Autodesk Inventor part; units mm, degrees
ref_plane "YZ Plane" through (0, 0, 0) normal (1, 0, 0) x (0, 1, 0)
ref_plane "XZ Plane" through (0, 0, 0) normal (0, 1, 0) x (-1, 0, 0)
ref_plane "XY Plane" through (0, 0, 0) normal (0, 0, 1) x (1, 0, 0)
sketch "Sketch1" plane through (0, 0, 0) normal (0, 1, 0) x (-1, 0, 0)
  line L0 (10, 22.5) -> (-10, 22.5)
  line L1 (-10, 22.5) -> (-10, -22.5)
  line L2 (-10, -22.5) -> (10, -22.5)
  line L3 (10, -22.5) -> (10, 22.5)
  line L4 (10, 22.5) -> (-10, -22.5) construction
  line L5 (-10, 22.5) -> (10, -22.5) construction
  line L6 (13.4184, 10.4917) -> (6.5816, 10.4917)
  line L7 (6.5816, 10.4917) -> (6.5816, -10.4917)
  line L8 (6.5816, -10.4917) -> (13.4184, -10.4917)
  line L9 (13.4184, -10.4917) -> (13.4184, 10.4917)
  line L10 (13.4184, 10.4917) -> (6.5816, -10.4917) construction
  line L11 (6.5816, 10.4917) -> (13.4184, -10.4917) construction
  line L12 (8.5, 21) -> (-8.5, 21)
  line L13 (-8.5, 21) -> (-8.5, -21)
  line L14 (-8.5, -21) -> (8.5, -21)
  line L15 (8.5, -21) -> (8.5, 21)
  line L16 (8.5, 21) -> (-8.5, -21) construction
  line L17 (-8.5, 21) -> (8.5, -21) construction
  circle A0 centre (8.5, 21) radius 0.75
  circle A1 centre (8.5, -21) radius 0.75
  circle A2 centre (-8.5, -21) radius 0.75
  circle A3 centre (-8.5, 21) radius 0.75
  point P0 (0, 0)
  point P1 (10, 0)
  point P2 (10, 10.4917)
  point P3 (10, -10.4917)
  dimension "d0" = 20
  dimension "d1" = 45
  dimension "d2" = 17
  dimension "d3" = 42
  dimension "d4" = 1.5
  dimension "d5" = 1.5
  dimension "d6" = 1.5
  dimension "d7" = 1.5
extrude "Extrusion1" add sketch "Sketch1" along normal blind 2 contours L3 L6 L15 A0 L12 A3 L13 A2 L14 A1 L8 L2 L1 L0 | L6 L7 L8 L15 A1 L14 A2 L13 A3 L12 A0
sketch "Sketch2" plane through (0, 0, 0) normal (0, -1, 0) x (1, 0, 0)
  line L0 (10, -22.5) -> (-10, -22.5)
  line L1 (10, -22.5) -> (13, -22.5)
  line L2 (13, -22.5) -> (13, 22.5)
  line L3 (-10, 22.5) -> (10, 22.5)
  line L4 (13, 22.5) -> (10, 22.5)
  line L5 (10, 22.5) -> (10, -22.5)
  point P0 (0, 0)
  dimension "d10" = 3
  dimension "d11" = 45
extrude "Extrusion2" add sketch "Sketch2" along normal blind 10 and the other way blind 2
fillet "Fillet1" radius 2 1 edges at (10, 0, 0)
sketch "Sketch3" plane through (13, -10, 22.5) normal (1, 0, 0) x (0, 0, -1)
  line L0 (0, 0) -> (45, 0)
  line L1 (22.5, 0) -> (22.5, 5)
  line L2 (22.5, 5) -> (22.5, 6)
  line L3 (22.5, 6) -> (7.5, 6)
  line L4 (7.5, 6) -> (37.5, 6)
  circle A0 centre (37.5, 6) radius 1.5
  circle A1 centre (7.5, 6) radius 1.5
  point P0 (22.5, 10)
  dimension "d17" = 5
  dimension "d18" = 1
  dimension "d19" = 15
  dimension "d20" = 30
  dimension "d21" = 3
  dimension "d22" = 3
extrude "Extrusion3" cut sketch "Sketch3" against normal blind 10
properties part number "Ultrasonic_holder"
Work out the finished part from the listing and answer in its coordinate system (mm). A direction names the side the tool comes from. Coordinates: 2 decimals unless noted, no trailing zeros. Order: outer loops, then holes, each group sorted by start corner. A loop starts at its lowest first (then second) coordinate and runs counter-clockwise, first axis right, second up. Notation, with made-up numbers: M -16.5,40 L 22.5,40 A9 cw 22.5,47 Z; hole C 39,-31 d4. An arc over 180 degrees is marked long. Use CSV: the item, a comma, the result in double quotes.
1) Flat-ended cylindrical pins translate along their axes: pin 1 Ø1.4 at (x, z) = (-8.5, -21) entering from +Y; pin 2 Ø6 at (y, z) = (-1.5, 14) entering from -X; pin 3 Ø5 at (y, z) = (-6, 3.5) entering from -X; pin 4 Ø2 at (y, z) = (0.5, 3.5) entering from -X. Find the tip coordinate at first contact, or state that the pin passes through.
Worked out:
pin 1,"passes through"
pin 2,"stops at x = -10"
pin 3,"stops at x = 10"
pin 4,"stops at x = -6.58"
2) For faces 4 (the face through (-8, 1, -10.492)), 5 (the face through (13, -4, 0)), 6 (the face through (-1, 0, 0)), determine the directions among +Z, -Z, +X, -X, +Y, -Y from which every point of the face is accessible in a straight line to the end or side of a thin tool.
Worked out:
face 4,"-X, +Y, -Y"
face 5,"+Z, -Z, +X, +Y, -Y"
face 6,"+Z, -Z, -X, -Y"
3) Consider line 1 (Z direction, x = -8.5, y = 0.55); line 2 (X direction, y = 1.5, z = 21); line 3 (Y direction, x = 12, z = -15). Determine where each line is inside the solid, lowest interval first. Write a range as [from, to].
Worked out:
line 1,"z = [-22.5, -21.75], [-20.25, -10.49], [10.49, 20.25], [21.75, 22.5]"
line 2,"x = [-10, -9.25], [-7.75, 7.75], [9.25, 13]"
line 3,"y = [-10, -5.5], [-2.5, 2]"
4) Section A-A on z = 15 is taken. Write down the section's boundary in (x, y), plus the area to 3 significant figures.
Worked out:
outline,"M -10,0 L 8,0 A2 cw 10,-2 L 10,-2.5 L 13,-2.5 L 13,2 L -10,2 Z; M 10,-10 L 13,-10 L 13,-5.5 L 10,-5.5 Z"
area,"67.9 mm^2"
5) Section D-D on y = -4 is taken. Write down the section's boundary in (x, z), plus the area to 3 significant figures.
Worked out:
outline,"M 10,-22.5 L 13,-22.5 L 13,-16.5 L 10,-16.5 Z; M 10,-13.5 L 13,-13.5 L 13,13.5 L 10,13.5 Z; M 10,16.5 L 13,16.5 L 13,22.5 L 10,22.5 Z"
area,"117 mm^2"
6) Section B-B on x = -8.5 is taken. Write down the section's boundary in (y, z).
Worked out:
outline,"M 0,-22.5 L 2,-22.5 L 2,-21.75 L 0,-21.75 Z; M 0,-20.25 L 2,-20.25 L 2,-10.49 L 0,-10.49 Z; M 0,10.49 L 2,10.49 L 2,20.25 L 0,20.25 Z; M 0,21.75 L 2,21.75 L 2,22.5 L 0,22.5 Z"
7) Section C-C on z = 21 is taken. Write down the section's boundary in (x, y).
Worked out:
outline,"M -10,0 L -9.25,0 L -9.25,2 L -10,2 Z; M -7.75,0 L 7.75,0 L 7.75,2 L -7.75,2 Z; M 9.25,-0.44 A2 cw 10,-2 L 10,-10 L 13,-10 L 13,2 L 9.25,2 Z"
8) Determine the mould class of faces 1 (the face through (-8.337, 0.986, -20.268)), 2 (the face through (-10, 1, 16)), 3 (the face through (11, -10, 0)) for opening direction X: released by +X, released by -X, zero draft, split by the parting line, or undercut.
Worked out:
face 1,"undercut"
face 2,"released by -X"
face 3,"zero draft"
